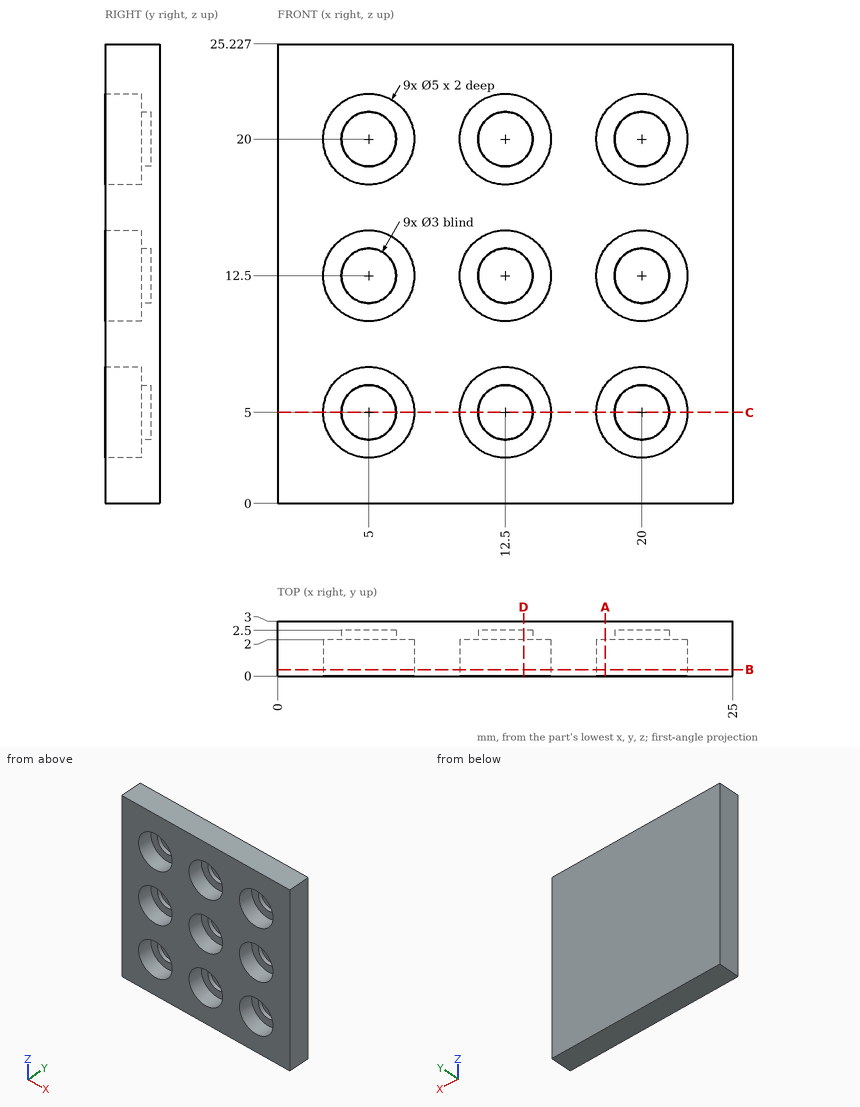
Can you work these out from the drawing? Everything is in mm from the part's minimum corner. Round coordinates to 2 decimals unless told otherwise and drop trailing zeros. Order: outer loops, then holes, each group sorted by start corner. A loop starts at its lowest first (then second) coordinate and runs counter-clockwise, first axis right, second up.
(1) If I drill on L1, parallel to Z at x = 7, y = 0.3 (1 decimal); L2, parallel to X at y = 2.3, z = 12.5; L3, parallel to X at y = 0.6, z = 20, over which ranges is the centre line in solid material (lowest first)?
Results are:
L1: z = 0 to 3.5, 6.5 to 11, 14 to 18.5, 21.5 to 25.2
L2: x = 0 to 3.5, 6.5 to 11, 14 to 18.5, 21.5 to 25
L3: x = 0 to 2.5, 7.5 to 10, 15 to 17.5, 22.5 to 25
(2) If we section it at B-B (y = 0.35): Count the separate pieces of the cut face and the enclosed holes in it, plus the area to 3 significant figures.
Results are:
separate pieces: 1
enclosed holes: 9
area: 454 mm2
(3) If we section it at D-D (x = 13.5): Please give me the cut outline in (y, z).
Results are:
outline: (0, 0) - (3, 0) - (3, 25.23) - (0, 25.23) - (0, 22.29) - (2, 22.29) - (2, 21.12) - (2.5, 21.12) - (2.5, 18.88) - (2, 18.88) - (2, 17.71) - (0, 17.71) - (0, 14.79) - (2, 14.79) - (2, 13.62) - (2.5, 13.62) - (2.5, 11.38) - (2, 11.38) - (2, 10.21) - (0, 10.21) - (0, 7.29) - (2, 7.29) - (2, 6.12) - (2.5, 6.12) - (2.5, 3.88) - (2, 3.88) - (2, 2.71) - (0, 2.71) - close
(4) I'm going to push flat-ended pins straight in: pin 1 (1.5 mm diameter, centred on x = 5, z = 21, fed in from -Y); pin 2 (1.8 mm diameter, centred on x = 5, z = 5, fed in from -Y). Where does each tip first touch, or does it pass through?
Results are:
pin 1: stops at y = 2
pin 2: stops at y = 2.5
(5) If we section it at A-A (x = 18): Please give me the cut outline in (y, z).
Results are:
outline: (0, 0) - (3, 0) - (3, 25.23) - (0, 25.23) - (0, 21.5) - (2, 21.5) - (2, 18.5) - (0, 18.5) - (0, 14) - (2, 14) - (2, 11) - (0, 11) - (0, 6.5) - (2, 6.5) - (2, 3.5) - (0, 3.5) - close
(6) If we section it at C-C (z = 5): Please give me the cut outline in (x, y).
Results are:
outline: (0, 0) - (2.5, 0) - (2.5, 2) - (3.5, 2) - (3.5, 2.5) - (6.5, 2.5) - (6.5, 2) - (7.5, 2) - (7.5, 0) - (10, 0) - (10, 2) - (11, 2) - (11, 2.5) - (14, 2.5) - (14, 2) - (15, 2) - (15, 0) - (17.5, 0) - (17.5, 2) - (18.5, 2) - (18.5, 2.5) - (21.5, 2.5) - (21.5, 2) - (22.5, 2) - (22.5, 0) - (25, 0) - (25, 3) - (0, 3) - close
